Read the model definition and answer for the solid it produces. Units are mm, in the model's axes. A direction names the side the tool comes from. Coordinates: 2 decimals unless noted, no trailing zeros. Loops run counter-clockwise (first coordinate to the right, second up) from the corner with the lowest first, then second, coordinate; pieces in that order, holes last. Notation, with made-up numbers: M 53.25,-16.75 L 60.25,-16.75 A11 ccw 60.25,2.25 Z; hole C 78.25,18.25 d2. An arc over 180 degrees is marked long. Use one line per item in the form item = value. Start each with the question number.
1. Find the intervals of material crossed by probe 1 along X at (y, z) = (2, -10); probe 2 along Z at (x, y) = (4, 3.75); probe 3 along Y at (x, z) = (-61, -4.5), in increasing order. Write a range as [from, to].
2. The part is cut by section B-B (z = -1.25). Give the vertices of the cut face in (x, y).
3. A flat-ended cylindrical pin translates along its axis: pin 1 (6 mm diameter, centred on x = -10.5, z = -10.5, fed in from -Y). Find the tip coordinate at first contact, or state that the pin passes through.
4. The part is cut by section A-A (y = -0.75). Give the vertices of the cut face in (x, z).
5. For a pull along X with two mould halves and no side action, classify faces 1 (the flat face through (68.58, 1, 0)), 2 (the flat face through (-68.58, 1, 0)), 3 (the flat face through (-10, -3.81, 12)), 4 (the flat face through (66.04, 0, 0)) as released by +X, released by -X, zero draft, split by the parting line, or undercut.
6. A tool of negligible diameter and unlimited length cuts with its end or side. For faces 5 (the flat face through (-1, 3.81, 0)), 6 (the flat face through (-1, 1, -13.97)), from which of +Z, -Z, +X, -X, +Y, -Y can it reach the whole face along a straight path? Write none if from no direction.
7. The part is cut by section C-C (x = -28.5). Give the vertices of the cut face in (y, z), plus the area to 3 significant figures.
from build123d import *

# Parameters (mm, degrees)
F0_W     = 132.08
F0_H     = 22.86
F1_DEPTH = 3.81
F2_T     = 2.54


with BuildPart() as f1:
    # F0 (on Front) → F1 (new body, symmetric)
    with BuildSketch(Plane.XZ):
        Rectangle(F0_W, F0_H)
    extrude(amount=F1_DEPTH, both=True)

    # F2
    f2_openings = [f1.faces().sort_by_distance(p)[0] for p in [
        (0, -3.81, 0),
    ]]
    offset(amount=F2_T, openings=f2_openings, kind=Kind.INTERSECTION)


solid = f1.part
Computed values:
q1.probe_1 = [-68.58, -66.04], [66.04, 68.58]
q1.probe_2 = [-13.97, -11.43], [11.43, 13.97]
q1.probe_3 = [3.81, 6.35]
q2.outline = M -68.58,-3.81 L -66.04,-3.81 L -66.04,3.81 L 66.04,3.81 L 66.04,-3.81 L 68.58,-3.81 L 68.58,6.35 L -68.58,6.35 Z
q3.pin_1 = -3.81
q4.outline = M -68.58,-13.97 L 68.58,-13.97 L 68.58,13.97 L -68.58,13.97 Z; hole M -66.04,-11.43 L 66.04,-11.43 L 66.04,11.43 L -66.04,11.43 Z
q5.face_1 = released by +X
q5.face_2 = released by -X
q5.face_3 = zero draft
q5.face_4 = undercut
q6.face_5 = -Y
q6.face_6 = -Z, +X, -X, +Y, -Y
q7.outline = M -3.81,-13.97 L 6.35,-13.97 L 6.35,13.97 L -3.81,13.97 L -3.81,11.43 L 3.81,11.43 L 3.81,-11.43 L -3.81,-11.43 Z
q7.area = 110 mm²
